Geometry check sheet. Reference: drawing and pictorial views, mm from the part's lowest x, y, z. Coordinates: 2 decimals unless noted, no trailing zeros. Loops run counter-clockwise (first coordinate to the right, second up) from the corner with the lowest first, then second, coordinate; pieces in that order, holes last. Notation, with made-up numbers: (-26, 4) -> (-4, 4) arc R36 cw to (-4, 43) -> close; hole circle Ø1 at (-24, 15.25). An arc over 180 degrees is marked (long way). Answer as a JSON object with one key per item and string values.
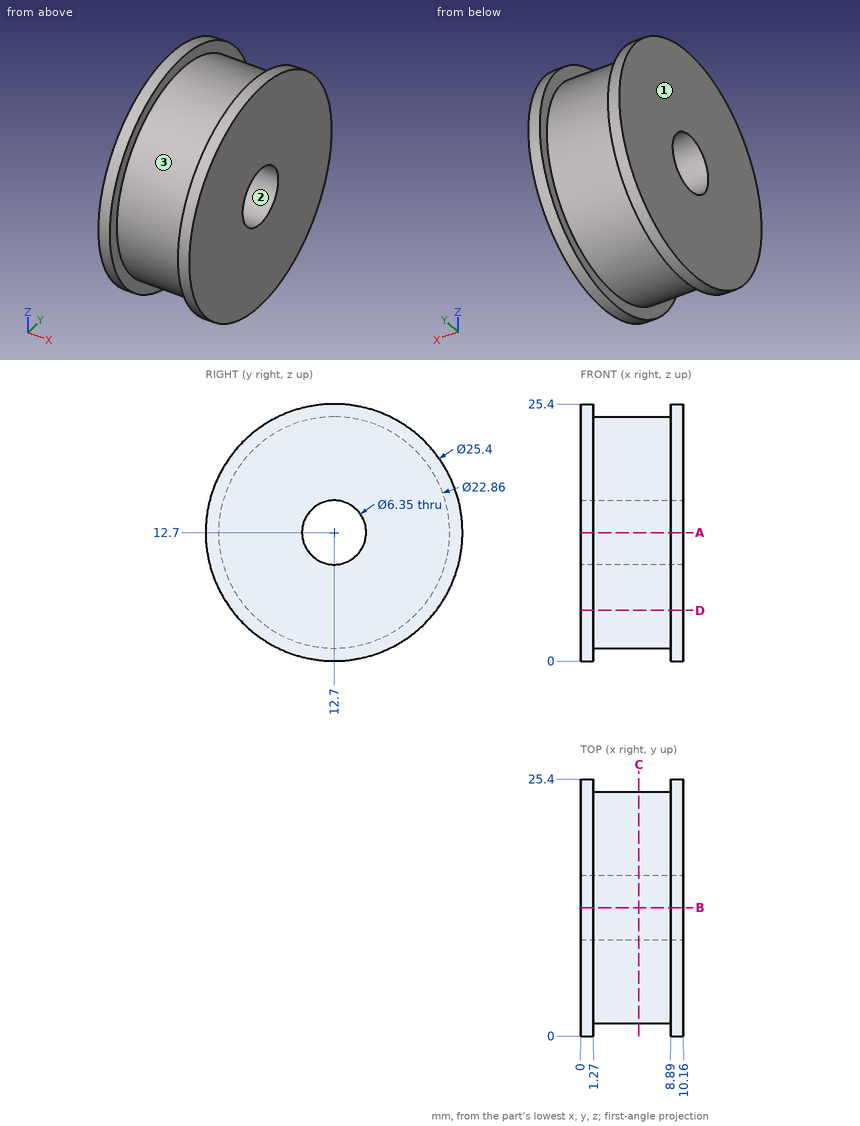
1. Mould release check, pull along Z, two halves, no side actions. Record for the marked faces 1, 2 and 3: released by +Z, released by -Z, zero draft, split by the parting line, or undercut.
Evaluation:
{"face 1": "zero draft", "face 2": "undercut", "face 3": "split by the parting line"}
2. Section check D-D, the plane z = 5. Record the boundary of the cut face in (x, y), then the cut area to 3 significant figures.
Evaluation:
{"outline": "(0, 2.6) -> (1.27, 2.6) -> (1.27, 4.25) -> (8.89, 4.25) -> (8.89, 2.6) -> (10.16, 2.6) -> (10.16, 22.8) -> (8.89, 22.8) -> (8.89, 21.15) -> (1.27, 21.15) -> (1.27, 22.8) -> (0, 22.8) -> close", "area": "180 mm^2"}
3. Depth check by flat-ended pin: P1, Ø4, axis at x = 1.5, z = 4, coming from the -Y side; P2, Ø3, axis at x = 2, y = 5.5, coming from the +Z side; P3, Ø4, axis at x = 5.5, y = 14, coming from the +Z side; P4, Ø5.5, axis at y = 12.7, z = 12.7, coming from the -X side. Enter the tip coordinate at first touch or a pass-through.
Evaluation:
{"P1": "stops at y = 1.92", "P2": "stops at z = 23.95", "P3": "stops at z = 24.13", "P4": "passes through"}
4. Section check A-A, the plane z = 12.7. Record the boundary of the cut face in (x, y) (3 decimals), then the cut area to 3 significant figures.
Evaluation:
{"outline": "(0, 0) -> (1.27, 0) -> (1.27, 1.27) -> (8.89, 1.27) -> (8.89, 0) -> (10.16, 0) -> (10.16, 9.525) -> (0, 9.525) -> close; (0, 15.875) -> (10.16, 15.875) -> (10.16, 25.4) -> (8.89, 25.4) -> (8.89, 24.13) -> (1.27, 24.13) -> (1.27, 25.4) -> (0, 25.4) -> close", "area": "174 mm^2"}
5. Thickness scan on probe 1 along Y at (x, z) = (7, 12.7) (3 decimals); probe 2 along X at (y, z) = (19.25, 2.5); probe 3 along Y at (x, z) = (8.5, 12). Record the ranges inside material, lowest first. Write a range as from..to.
Evaluation:
{"probe 1": "y = 1.27..9.525, 15.875..24.13", "probe 2": "x = 0..1.27, 8.89..10.16", "probe 3": "y = 1.29..9.6, 15.8..24.11"}
6. Section check C-C, the plane x = 5.75. Record the boundary of the cut face in (y, z) (3 decimals), then the cut area to 3 significant figures.
Evaluation:
{"outline": "circle Ø22.86 at (12.7, 12.7); hole circle Ø6.35 at (12.7, 12.7)", "area": "379 mm^2"}
